Can you work these out from the drawing? Everything is in mm from the part's minimum corner. Coordinates: 2 decimals unless noted, no trailing zeros. Write each loop counter-clockwise with the first axis right and the second up, starting at its lowest first coordinate (ties: lowest second). Pieces come first, ordered by that corner, then holes. Notation, with made-up numbers: (67, 33.5) -> (114, 33.5) arc R22 ccw to (114, 72.5) -> close; hole circle Ø3 at (1.5, 67.5). An arc over 180 degrees is marked (long way). Use a Markdown table: item, result. Add a question column.
Item 1: If I drill on line 1 along Y through (x, z) = (16, 18.5); line 2 along X through (y, z) = (79, 13); line 3 along X through (y, z) = (83, 9.5), over which ranges is the centre line in solid material (lowest first)? Write a range as from..to.
Item 2: Imagine slicing it at C-C, the plane y = 3.5. Write out the boundary of the cut face in (x, z), and give its area (4 significant figures).
Item 3: Imagine slicing it at A-A, the plane x = 106.5. Write out the boundary of the cut face in (y, z), and give its area (4 significant figures).
Item 4: Imagine slicing it at B-B, the plane y = 83. Write out the boundary of the cut face in (x, z).
Item 5: If we mould it in two halves opening along Z, with no side actions, what happens to the marked faces 1, 2 and 3? For each: pulls with the +Z half, pulls with the -Z half, needs draft (parallel to the pull), parting line crosses it, or undercut.
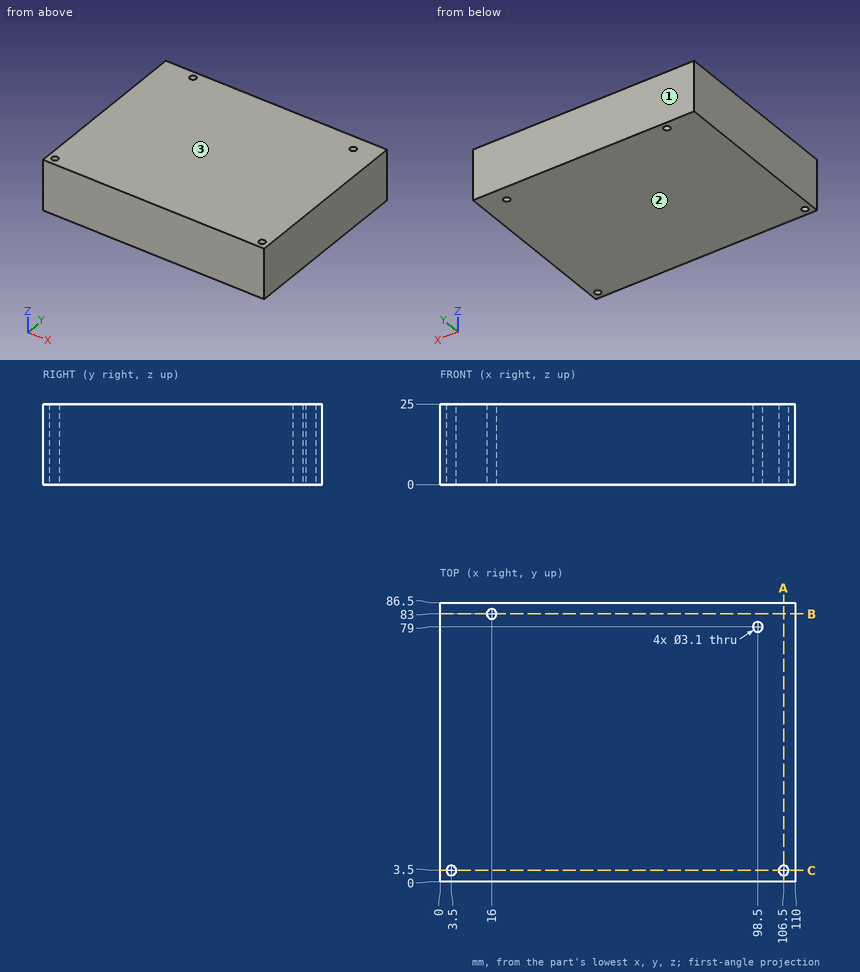
Ans:
| question | item | result |
|---|---|---|
| 1 | line 1 | y = 0..81.45, 84.55..86.5 |
| 1 | line 2 | x = 0..96.95, 100.05..110 |
| 1 | line 3 | x = 0..14.45, 17.55..110 |
| 2 | outline | (0, 0) -> (1.95, 0) -> (1.95, 25) -> (0, 25) -> close; (5.05, 0) -> (104.95, 0) -> (104.95, 25) -> (5.05, 25) -> close; (108.05, 0) -> (110, 0) -> (110, 25) -> (108.05, 25) -> close |
| 2 | area | 2,595 mm^2 |
| 3 | outline | (0, 0) -> (1.95, 0) -> (1.95, 25) -> (0, 25) -> close; (5.05, 0) -> (86.5, 0) -> (86.5, 25) -> (5.05, 25) -> close |
| 3 | area | 2,085 mm^2 |
| 4 | outline | (0, 0) -> (14.45, 0) -> (14.45, 25) -> (0, 25) -> close; (17.55, 0) -> (110, 0) -> (110, 25) -> (17.55, 25) -> close |
| 5 | face 1 | needs draft |
| 5 | face 2 | pulls with the -Z half |
| 5 | face 3 | pulls with the +Z half |
